Geometry: final body of the model. Coordinates: model frame, mm. A direction names the side the tool comes from. Coordinates: 2 decimals unless noted, no trailing zeros. Order: outer loops, then holes, each group sorted by start corner. A loop starts at its lowest first (then second) coordinate and runs counter-clockwise, first axis right, second up. Notation, with made-up numbers: (71, 63) -> (124, 63) arc R26 ccw to (124, 80) -> close; hole circle Ø11 at (46, 68). An arc over 180 degrees is marked (long way). Use one line per item in the form item = value.
Autodesk Inventor part; units mm, degrees
ref_plane "Work Plane1" through (-3.25, 0, -23.5) normal (0, 0, -1) x (-1, 0, 0)
ref_plane "YZ Plane" through (0, 0, 0) normal (1, 0, 0) x (0, 1, 0)
ref_plane "XZ Plane" through (0, 0, 0) normal (0, 1, 0) x (-1, 0, 0)
sketch "Sketch1" plane through (0, 0, 0) normal (0, 1, 0) x (-1, 0, 0)
  line L0 (8.25, -7) -> (-1.75, -7)
  line L1 (-1.75, -7) -> (-1.75, -18.5)
  line L2 (3.25, -23.5) -> (3.25, -23.5)
  line L3 (8.25, -18.5) -> (8.25, -7)
  line L4 (6.5, 0) -> (0, 0)
  line L5 (0, 0) -> (0, -7)
  line L6 (0, -7) -> (6.5, -7)
  line L7 (6.5, -7) -> (6.5, 0)
  line L8 (3.25, -4.5122) -> (3.25, -12.4364) construction
  arc A0 (3.25, -23.5) -> (8.25, -18.5) centre (3.25, -18.5) ccw
  arc A1 (-1.75, -18.5) -> (3.25, -23.5) centre (3.25, -18.5) ccw
  line L9 (3.25, -23.5) -> (3.25, -30.5)
  line L10 (3.25, -30.5) -> (3.25, -45.2683) construction
  line L11 (3.25, -45.2683) -> (8.7503, -49.7156) construction
  spline S0 degree 2 poles (3.25, -30.5) (3.25, -45.2683) (8.7503, -49.7156) knots 1 1 1 2 2 2
  point P0 (8.25, -23.5)
  dimension "d0" = 10
  dimension "d1" = 6.5
  dimension "d3" = 16.5
  dimension "d4" = 5
  dimension "d5" = 7
  dimension "d15" = 7
extrude "Extrusion1" add sketch "Sketch1" along normal mid plane 7.5 contours L3 A0 A1 L1 L0
extrude "Extrusion2" add sketch "Sketch1" along normal mid plane 3 contours L0 L5 L4 L7
ref_plane "Work Plane1" through (-3.25, 0, -23.5) normal (0, 0, -1) x (-1, 0, 0)
sketch "Sketch2" plane through (-3.25, 0, -23.5) normal (0, 0, -1) x (-1, 0, 0)
  circle A0 centre (0, 0) radius 3.75
  point P0 (-3.25, 0)
  dimension "d12" = 7.5
extrude "Extrusion3" add sketch "Sketch2" along normal blind 7 and the other way blind 2
sketch "Sketch3" plane through (-3.25, 0, -30.5) normal (0, 0, -1) x (-1, 0, 0)
  circle A0 centre (0, 0) radius 2.75
  point P0 (-3.25, 0)
  dimension "d18" = 5.5
sweep "Sweep1" add profiles "Sketch3" path "Sketch1" path curves L9 S0
properties part number "USB_cable"
1) Material intervals for probe 1 along Y at (x, z) = (-3, -25.5); probe 2 along X at (y, z) = (2.5, -16); probe 3 along Z at (x, y) = (-7, -3), sorted ascending. Write a range as from..to.
Results found:
probe_1 = -3.74..3.74
probe_2 = -8.25..1.75
probe_3 = -21.81..-7
2) Contact query for flat-ended pins moving along their axis: P1, Ø3, axis at x = -7.5, y = 2.5, coming from the +Z side; P2, Ø2, axis at x = -3.5, z = -3, coming from the -Y side; P3, Ø2.5, axis at y = 0, z = -3, coming from the -X side; P4, Ø1.5, axis at x = -3.5, y = 1, coming from the -Z side. Output: stop coordinate, or through.
Results found:
P1 = 0
P2 = -1.5
P3 = -6.5
P4 = -48.43
3) Access query for faces 1 (the cylindrical face through (-6.714, 1.436, -26.093)), 2 (the flat face through (-3, -1.5, -3)), 3 (the cylindrical face through (-7.804, -0.053, -20.563)). Directions: +Z, -Z, +X, -X, +Y, -Y. A direction counts if a zero-diameter tool reaches every point of the face in a straight line with its end or side. Return the directions, or none.
Results found:
face_1 = none
face_2 = +Z, +X, -X, -Y
face_3 = -X
4) Section A-A, the plane x = 1.25. Output: boundary loops of the cut face in (y, z).
Results found:
outline = (-3.75, -20.68) -> (3.75, -20.68) -> (3.75, -7) -> (-3.75, -7) -> close
5) Pull-direction query (Z, two-part tool) for faces 4 (the flat face through (-8.69, -0.02, -49.79)), 5 (the flat face through (0, 0, -3)), 6 (the flat face through (-2, 3, -30.5)); classes: released by +Z, released by -Z, zero draft, split by the parting line, or undercut.
Results found:
face_4 = released by -Z
face_5 = zero draft
face_6 = undercut
